Could you check a few things on this model? Use its own coordinates, in mm. A direction names the side the tool comes from. Round coordinates to 2 decimals unless told otherwise and drop trailing zeros. Write each loop counter-clockwise with the first axis right and the second up, starting at its lowest first coordinate (ties: lowest second). Pieces come first, ordered by that corner, then holes. Notation, with made-up numbers: M -8,28 L 3,28 A17 ccw 3,55 Z; hole C 53.5,79 d1. An arc over 180 degrees is marked long. One line per question, with ' | ' between items. Start each with the question number.
```python
from build123d import *

# Parameters (mm, degrees)
F1_DEPTH = 3.175
F2_R     = 1.5875
F3_DEPTH = 3.175


with BuildPart() as f1:
    # F0 (on Front) → F1 (new body)
    with BuildSketch(Plane.XZ):
        with BuildLine():
            ThreePointArc((-2.396699, -12.471802), (8.088632, -9.791018), (12.7, 0))
            ThreePointArc((12.7, 0), (8.089103, 9.790629), (-2.395498, 12.472032))
            ThreePointArc((-2.395498, 12.472032), (-12.7, 0.000611), (-2.396699, -12.471802))
        make_face()
        with BuildLine():
            ThreePointArc((-2.396699, -12.471802), (-12.7, 0.000611), (-2.395498, 12.472032))
            Line((-2.395498, 12.472032), (-50.8, 3.175))
            ThreePointArc((-50.8, 3.175), (-48.554936, 2.245064), (-47.625, 0))
            ThreePointArc((-47.625, 0), (-48.546238, -2.236332), (-50.775351, -3.174904))
            Line((-50.775351, -3.174904), (-2.396699, -12.471802))
        make_face()
        with BuildLine():
            ThreePointArc((-47.625, 0), (-48.554936, 2.245064), (-50.8, 3.175))
            ThreePointArc((-50.8, 3.175), (-53.974976, -0.012325), (-50.775351, -3.174904))
            ThreePointArc((-50.775351, -3.174904), (-48.546238, -2.236332), (-47.625, 0))
        make_face()
    extrude(amount=F1_DEPTH)

    # F2 (on face) → F3 (join)
    with BuildSketch(Plane.XZ.offset(3.175)):
        with Locations((-50.8, 0)):
            Circle(F2_R)
    extrude(amount=F3_DEPTH)


solid = f1.part
```
1. Which directions (+Z, -Z, +X, -X, +Y, -Y) give clear straight access to the entire face, cutting with the end or side of a thin tool? Please do faces 1 (the face through (-14, 0, 0)), 2 (the face through (-52.386, -4.74, 0.07)).
2. Suppose I cut it at B-B (x = -28). Write out the boundary of the cut face in (y, z) (3 decimals), and give its area (3 significant figures).
3. I need wall thicknesses on line 1 along Y through (x, z) = (-5, -11) (3 decimals); line 2 along X through (y, z) = (-2.5, 0.25); line 3 along Z through (x, y) = (3, -1.5). Which ranges of each line are inside material? Lowest first, please. Write a range as from..to.
4. Suppose I cut it at C-C (z = -10.75). Write out the boundary of the cut face in (x, y) (3 decimals), and give its area (3 significant figures).
5. I'm going to push flat-ended pins straight in: P1, Ø1, axis at x = -47, y = -2, coming from the -Z side; P2, Ø4, axis at x = 3, z = 7, coming from the -Y side (3 decimals); P3, Ø1, axis at x = 4, y = -2.5, coming from the +Z side. Where does each tip first touch, or does it pass through?
Computed:
1) face 1: +Z, -Z, +X, -X, +Y | face 2: -Y
2) outline: M -3.175,-7.552 L 0,-7.552 L 0,7.554 L -3.175,7.554 Z | area: 48.0 mm²
3) line 1: y = -3.175..0 | line 2: x = -53.97..12.7 | line 3: z = -12.34..12.34
4) outline: M -11.357,-3.175 L 6.762,-3.175 L 6.762,0 L -11.357,0 Z | area: 57.5 mm²
5) P1: stops at z = -4 | P2: stops at y = -3.175 | P3: stops at z = 12.21
